```python
from build123d import *

# Parameters (mm, degrees)
F0_W     = 12
F0_H     = 12
F0_R     = 1.5
F1_DEPTH = 3
F2_W     = 12
F2_H     = 4
F3_DEPTH = 5
F5_R     = 2.99999
F6_DEPTH = 6


# Not quite as in the source:
# - a fillet or chamfer is up to 0.001 mm smaller than in the source, because OpenCascade refuses the exact size


with BuildPart() as f1:
    # F0 (on Top) → F1 (new body)
    with BuildSketch(Plane.XY):
        Rectangle(F0_W, F0_H)
        Circle(F0_R, mode=Mode.SUBTRACT)
    extrude(amount=F1_DEPTH)

    # F2 (on face) → F3 (join)
    with BuildSketch(Plane.XY.offset(3)):
        with Locations((0, 4)):
            Rectangle(F2_W, F2_H)
    extrude(amount=F3_DEPTH)

    # F5 (radius 3 in the source; OpenCascade refuses exactly that, so slightly less here)
    f5_edges = [f1.edges().sort_by_distance(p)[0] for p in [
        (0, -6, 3),
    ]]
    fillet(f5_edges, radius=F5_R)

    # F4 (on face) → F6 (cut)
    with BuildSketch(Plane.XY.offset(8)):
        with BuildLine():
            ThreePointArc((-2.8722813233, 2), (-1.0480971731, -3.3393850206), (3.5, 0))
            ThreePointArc((3.5, 0), (3.3393850206, 1.0480971731), (2.8722813233, 2))
            Line((2.8722813233, 2), (-2.8722813233, 2))
        make_face()
        with BuildLine():
            Line((-2.8722813233, 2), (2.8722813233, 2))
            ThreePointArc((2.8722813233, 2), (0, 3.5), (-2.8722813233, 2))
        make_face()
    extrude(amount=-F6_DEPTH, mode=Mode.SUBTRACT)


solid = f1.part
```
For this review, take the finished solid that the model builds, in its own axes (mm). A direction names the side the tool comes from. Give positions to 0.01 mm unless a question says otherwise; leave off trailing zeros. Write each loop counter-clockwise with the first axis right and the second up, starting at its lowest first coordinate (ties: lowest second). Pieces come first, ordered by that corner, then holes. Notation, with made-up numbers: M -34.5,-23.75 L -8.5,-23.75 A8 cw -8.5,-8.75 Z; hole C 62,54 d1. An arc over 180 degrees is marked long. One line per item, written item: value.
1) For faces 1 (the flat face through (0, -2, 2)), 2 (the flat face through (-6, 1, 2)), 3 (the flat face through (4, 0, 3)), list the 3-axis set-ups (+Z, -Z, +X, -X, +Y, -Y) from which the entire face can be reached by the end or side of a thin tool; tool diameter is ignored.
Results are:
face 1: +Z
face 2: +Z, -Z, -X, +Y, -Y
face 3: +Z, +X, -X, -Y
2) The part is to be moulded in two halves that separate along Y. For faces 4 (the flat face through (0, 6, 4)), 5 (the flat face through (1.2, 1.4, 0)), 6 (the cylindrical face through (-1.5, 0.07, 0.99)), say which applies: +Y half, -Y half, draft (parallel to the pull), parting line (faces both ways), or undercut.
Results are:
face 4: +Y half
face 5: draft
face 6: undercut
3) For line 1 (X direction, y = 0, z = 1.4); line 2 (Z direction, x = -3, y = -3); line 3 (Y direction, x = 3, z = 6.25), list the stretches that pass through material, from the lowest coordinate up. Write a range as from..to.
Results are:
line 1: x = -6..-1.5, 1.5..6
line 2: z = 0..3
line 3: y = 2..6
4) Take a section at D-D, the plane y = 3.25. Write out the cut boundary in (x, z).
Results are:
outline: M -6,0 L 6,0 L 6,8 L 1.3,8 L 1.3,2 L -1.3,2 L -1.3,8 L -6,8 Z
5) Take a section at C-C, the plane z = 6.5. Write out the cut boundary in (x, y).
Results are:
outline: M -6,2 L -2.87,2 A3.5 cw 2.87,2 L 6,2 L 6,6 L -6,6 Z
6) For P1, Ø2, axis at x = -3.5, y = 0.5, coming from the +Z side; P2, Ø3, axis at x = 3.5, z = 7, coming from the -Y side; P3, Ø4.5, axis at x = 5, y = 0.5, coming from the +Z side; P4, Ø5.5, axis at x = -0.5, y = -0.5, coming from the +Z side, all flat-tipped, find the tip position at first contact; note any pin that passes through.
Results are:
P1: stops at z = 3
P2: stops at y = 2
P3: stops at z = 8
P4: stops at z = 2
7) Take a section at A-A, the plane y = 0.25. Write out the cut boundary in (x, z).
Results are:
outline: M -6,0 L -1.48,0 L -1.48,2 L -3.49,2 L -3.49,3 L -6,3 Z; M 1.48,0 L 6,0 L 6,3 L 3.49,3 L 3.49,2 L 1.48,2 Z
